Model file for the job. Use its own axes, mm. A direction names the side the tool comes from. Round coordinates to 2 decimals unless told otherwise and drop trailing zeros. Order: outer loops, then holes, each group sorted by start corner. A loop starts at its lowest first (then second) coordinate and runs counter-clockwise, first axis right, second up. Notation, with made-up numbers: (19.5, -9) - (37.5, -9) arc R16 ccw to (37.5, 2) - close; hole circle Ø5 at (-6.75, 79.25). An arc over 180 degrees is marked (long way). Use one line per item in the form item = value.
from build123d import *

# Parameters (mm, degrees)
F2_DEPTH = 10
F3_DEPTH = 4.5
F5_D     = 8
F7_D     = 6.6


with BuildPart() as f2:
    # F0 (on Front) → F2 (new body, symmetric)
    with BuildSketch(Plane.XZ):
        with BuildLine():
            Line((4.7648381702, 12), (-10.5830052443, 12))
            ThreePointArc((-10.5830052443, 12), (-11.7765474066, -10.831109416), (11.0744966927, -11.5479661847))
            Line((11.0744966927, -11.5479661847), (4.7648381702, 12))
        make_face()
    extrude(amount=F2_DEPTH, both=True)

    # F1 (on Front) → F3 (cut, symmetric)
    with BuildSketch(Plane.XZ):
        Polygon((11.0744966927, 12), (-9, 12), (-16.5025773881, -16), (11.0744966927, -16), align=None)
    extrude(amount=F3_DEPTH, both=True, mode=Mode.SUBTRACT)

    # F5 (through all)
    with Locations(Plane.XZ.offset(10)):
        with Locations((2, 3)):
            Hole(F5_D / 2)

    # F7 (through all)
    with Locations(Plane.YZ):
        with Locations((0, 0)):
            Hole(F7_D / 2)


solid = f2.part
(1) Pin check, flat tips, straight feed: pin 1 (1.5 mm diameter, centred on y = 6, z = 5.5, fed in from -X); pin 2 (2 mm diameter, centred on x = 5.5, y = -7.5, fed in from -Z). Stop position of each tip, or through.
Report:
pin_1 = -15.28
pin_2 = -15.35
(2) Slice it at B-B on x = 1.5. Give the cut face in (y, z), then the cut area to 3 significant figures.
Report:
outline = (-10, -15.93) - (-4.5, -15.93) - (-4.5, -0.97) - (-10, -0.97) - close; (-10, 6.97) - (-4.5, 6.97) - (-4.5, 12) - (-10, 12) - close; (4.5, -15.93) - (10, -15.93) - (10, -0.97) - (4.5, -0.97) - close; (4.5, 6.97) - (10, 6.97) - (10, 12) - (4.5, 12) - close
area = 220 mm2
(3) Probe probe 1 along Y at (x, z) = (-12.75, 0); probe 2 along Y at (x, z) = (-1.25, -11.5); probe 3 along X at (y, z) = (-8.75, 5.5). List the from-to ranges inside material, lowest first. Write a range as [from, to].
Report:
probe_1 = [-10, -3.3], [3.3, 10]
probe_2 = [-10, -4.5], [4.5, 10]
probe_3 = [-15.02, -1.12], [5.12, 6.51]
(4) Tool access for faces 1 (the face through (-2, -4.5, -2)), 2 (the face through (-13.7, 0.43, 3.27)): list every direction of +Z, -Z, +X, -X, +Y, -Y with a clear straight run to the whole face (end or side of a thin tool).
Report:
face_1 = -Z, +X
face_2 = +X, -X
(5) Pull direction X, two halves, no side cores. Call faces 3 (the face through (-3, 10, -2)), 4 (the face through (-10.984, -0.063, 4.597)), 5 (the face through (2.867, -7.212, -0.905)): released by +X, released by -X, zero draft, split by the parting line, or undercut.
Report:
face_3 = zero draft
face_4 = released by +X
face_5 = undercut
(6) Slice it at D-D on z = 4.25. Give the cut face in (x, y), then the cut area to 3 significant figures.
Report:
outline = (-15.43, -10) - (-1.8, -10) - (-1.8, -4.5) - (-11.08, -4.5) - (-11.08, 4.5) - (-1.8, 4.5) - (-1.8, 10) - (-15.43, 10) - close; (5.8, -10) - (6.84, -10) - (6.84, -4.5) - (5.8, -4.5) - close; (5.8, 4.5) - (6.84, 4.5) - (6.84, 10) - (5.8, 10) - close
area = 200 mm2
(7) Slice it at A-A on z = -11. Give the cut face in (x, y), then the cut area to 3 significant figures.
Report:
outline = (-11.62, -10) - (10.93, -10) - (10.93, -4.5) - (-11.62, -4.5) - close; (-11.62, 4.5) - (10.93, 4.5) - (10.93, 10) - (-11.62, 10) - close
area = 248 mm2
(8) Slice it at C-C on y = -1.5. Give the cut face in (x, z), then the cut area to 3 significant figures.
Report:
outline = (-15.73, -2.94) arc R16 ccw to (-14.19, -7.38) - (-13, -2.94) - close; (-15.73, 2.94) - (-11.43, 2.94) - (-9, 12) - (-10.58, 12) arc R16 ccw to start
area = 39.3 mm2
